from build123d import *

# Parameters (mm, degrees)
BOSS_EXTRU_1_DEPTH            = 20
DIAM_TRE_DU_PER_AGE_5_0_5_1_D = 5
DIAM_TRE_DU_PER_AGE_5_0_5_2_D = 5


with BuildPart() as part:
    # Esquisse1 → Boss.-Extru.1 (new body, symmetric)
    with BuildSketch(Plane(origin=(0, 0, 0), x_dir=(0, 0, -1), z_dir=(1, 0, 0))):
        with BuildLine():
            Line((0, 55), (0, 4))
            ThreePointArc((0, 4), (1.171572875, 1.171572875), (4, 0))
            Line((4, 0), (55, 0))
            Line((55, 0), (55, 2))
            Line((55, 2), (4, 2))
            ThreePointArc((4, 2), (2.585786438, 2.585786438), (2, 4))
            Line((2, 4), (2, 55))
            Line((2, 55), (0, 55))
        make_face()
    extrude(amount=BOSS_EXTRU_1_DEPTH, both=True)

    # Diamètre du perçage Ø5.0 (5)1 (through all)
    with Locations(Plane(origin=(0, 2, 0), x_dir=(1, 0, 0), z_dir=(0, 1, 0))):
        with Locations((-10, 45), (-10, 25), (10, 35), (10, 15)):
            Hole(DIAM_TRE_DU_PER_AGE_5_0_5_1_D / 2)

    # Diamètre du perçage Ø5.0 (5)2 (through all)
    with Locations(Plane(origin=(0, 0, -2), x_dir=(-1, 0, 0), z_dir=(0, 0, -1))):
        with Locations((-10, 15), (-10, 35), (10, 25), (10, 45)):
            Hole(DIAM_TRE_DU_PER_AGE_5_0_5_2_D / 2)


solid = part.part
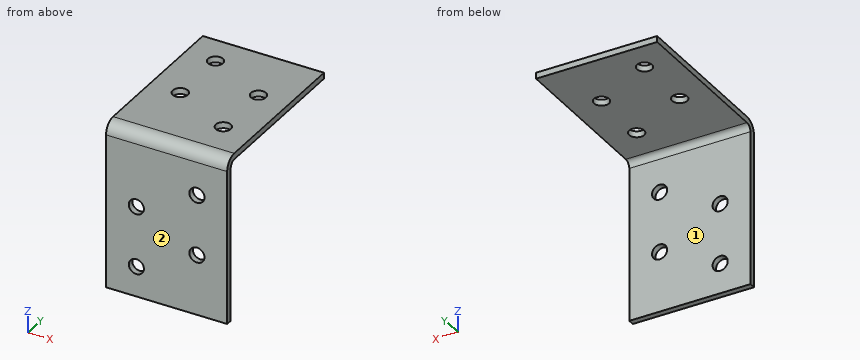
Model file for the job. Use its own axes, mm. Face numbers are marked on the shaded views. A direction names the side the tool comes from. Give positions to 0.01 mm unless a question says otherwise; leave off trailing zeros. Order: outer loops, then holes, each group sorted by start corner. A loop starts at its lowest first (then second) coordinate and runs counter-clockwise, first axis right, second up. Notation, with made-up numbers: (32, 85) - (50, 85) arc R13 cw to (50, 98) - close; hole circle Ø6 at (21, -16.5). An arc over 180 degrees is marked (long way). Write item = value, one per line. Start each with the question number.
1. Drop flat-ended pins along their axis: P1, Ø4, axis at x = 10, z = -15, coming from the +Y side; P2, Ø6.5, axis at x = 10, z = -35, coming from the +Y side; P3, Ø2, axis at x = 14.5, y = 14, coming from the -Z side. Give the stop position or say it passes through.
2. Probe line 1 along X through (y, z) = (1, -35); line 2 along X through (y, z) = (1.3, -25); line 3 along Z through (x, y) = (-10, 1). List the from-to ranges inside material, lowest first.
3. Cut at B-B, the plane z = -16.5. List the corners of the cut face in (x, y), and give its area (3 significant figures).
4. Cut at A-A, the plane y = 13.5. List the corners of the cut face in (x, z).
5. Cut at C-C, the plane x = -10. List the corners of the cut face in (y, z), and give its area (3 significant figures).
6. Cut at D-D, the plane x = -1.5. List the corners of the cut face in (y, z).
7. Which spindle directions (+Z, -Z, +X, -X, +Y, -Y) get a long thin tool onto all of the face, cutting with end or side? Do the marked faces 1 and 2. Say none if no direction does.
Taken from the geometry:
q1.P1 = through
q1.P2 = 2
q1.P3 = -2
q2.line_1 = -20 to 7.5, 12.5 to 20
q2.line_2 = -20 to -12.5, -7.5 to 20
q2.line_3 = -55 to -47.5, -42.5 to -27.5, -22.5 to -1.35
q3.outline = (-20, 0) - (8, 0) - (8, 2) - (-20, 2) - close; (12, 0) - (20, 0) - (20, 2) - (12, 2) - close
q3.area = 72.0 mm²
q4.outline = (-20, -2) - (8, -2) - (8, 0) - (-20, 0) - close; (12, -2) - (20, -2) - (20, 0) - (12, 0) - close
q5.outline = (0, -55) - (2, -55) - (2, -47.5) - (0, -47.5) - close; (0, -42.5) - (2, -42.5) - (2, -27.5) - (0, -27.5) - close; (0, -22.5) - (2, -22.5) - (2, -4) arc R2 cw to (4, -2) - (22.5, -2) - (22.5, 0) - (4, 0) arc R4 ccw to (0, -4) - close; (27.5, -2) - (42.5, -2) - (42.5, 0) - (27.5, 0) - close; (47.5, -2) - (55, -2) - (55, 0) - (47.5, 0) - close
q5.area = 173 mm²
q6.outline = (0, -55) - (2, -55) - (2, -4) arc R2 cw to (4, -2) - (55, -2) - (55, 0) - (4, 0) arc R4 ccw to (0, -4) - close
q7.face_1 = -Z, +X, -X, +Y
q7.face_2 = +Z, -Z, +X, -X, -Y
